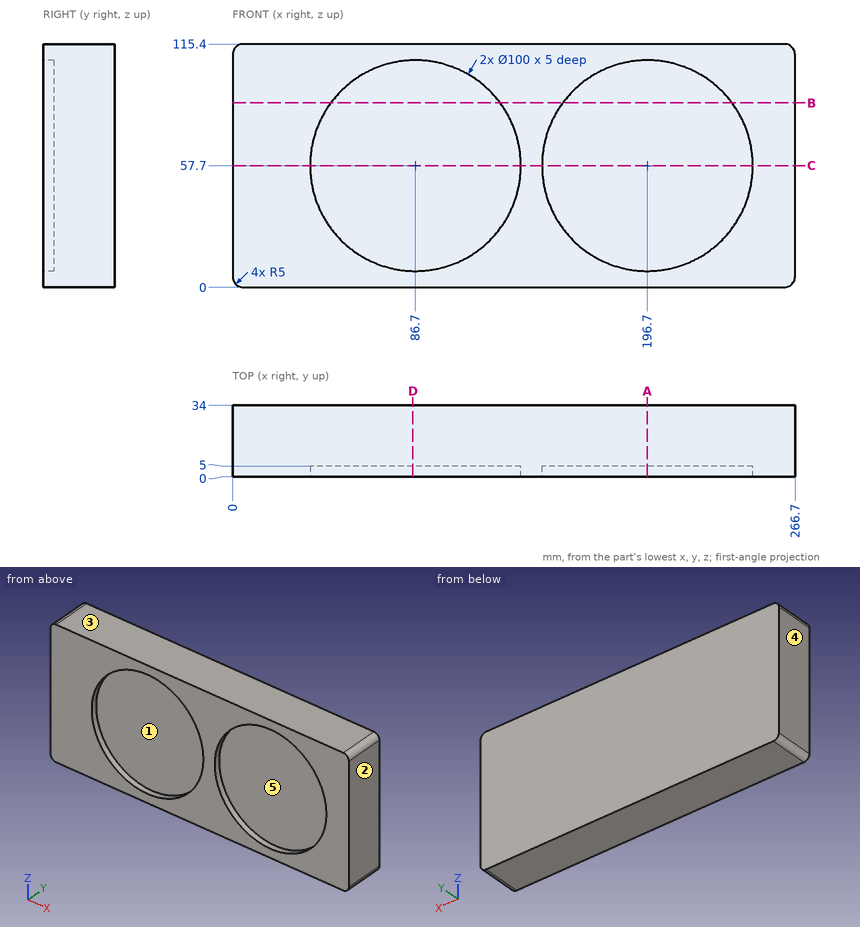
The drawing under review shows one solid part. Ordinate dimensions are in mm from its lowest x, y, z. A direction names the side the tool comes from. Coordinates: 2 decimals unless noted, no trailing zeros. Loops run counter-clockwise (first coordinate to the right, second up) from the corner with the lowest first, then second, coordinate; pieces in that order, holes last. Notation, with made-up numbers: (45, 88.5) - (67, 88.5) arc R23 cw to (67, 102.5) - close; hole circle Ø11 at (26.25, 74.5). An arc over 180 degrees is marked (long way). Return JSON: item names as keys, results as strings.
Item 1: Mouldability with a two-part tool opening along X and no side actions: class the marked faces 3, 4 and 5 as pulls with the +X half, pulls with the -X half, needs draft (parallel to the pull), parting line crosses it, or undercut.
Determined:
{"face 3": "needs draft", "face 4": "pulls with the -X half", "face 5": "undercut"}
Item 2: Insertion check: pin 1 (1 mm diameter, centred on x = 199.5, z = 103, fed in from -Y). The pin has a flat end and moves straight along its axis. Give the tip position at first contact, or say it passes through.
Determined:
{"pin 1": "stops at y = 5"}
Item 3: Take a section at A-A (x = 196.7). Give the boundary of the cut face in (y, z), then the cut area to 3 significant figures.
Determined:
{"outline": "(0, 0) - (34, 0) - (34, 115.4) - (0, 115.4) - (0, 107.7) - (5, 107.7) - (5, 7.7) - (0, 7.7) - close", "area": "3,420 mm2"}
Item 4: For the marked faces 1 and 2, list the 3-axis set-ups (+Z, -Z, +X, -X, +Y, -Y) from which the entire face can be reached by the end or side of a thin tool; tool diameter is ignored.
Determined:
{"face 1": "-Y", "face 2": "+Z, -Z, +X, +Y, -Y"}
Item 5: Take a section at D-D (x = 85.5). Give the boundary of the cut face in (y, z).
Determined:
{"outline": "(0, 0) - (34, 0) - (34, 115.4) - (0, 115.4) - (0, 107.69) - (5, 107.69) - (5, 7.71) - (0, 7.71) - close"}
Item 6: For line 1 (Z direction, x = 86, y = 1); line 2 (X direction, y = 1, z = 57); line 3 (Y direction, x = 54.5, z = 73.5), list the stretches that pass through material, from the lowest coordinate up.
Determined:
{"line 1": "z = 0 to 7.7, 107.7 to 115.4", "line 2": "x = 0 to 36.7, 136.7 to 146.7, 246.7 to 266.7", "line 3": "y = 5 to 34"}
Item 7: Take a section at C-C (z = 57.7). Give the boundary of the cut face in (x, y).
Determined:
{"outline": "(0, 0) - (36.7, 0) - (36.7, 5) - (136.7, 5) - (136.7, 0) - (146.7, 0) - (146.7, 5) - (246.7, 5) - (246.7, 0) - (266.7, 0) - (266.7, 34) - (0, 34) - close"}
Item 8: Take a section at B-B (z = 87.5). Give the boundary of the cut face in (x, y), then the cut area to 3 significant figures.
Determined:
{"outline": "(0, 0) - (46.55, 0) - (46.55, 5) - (126.85, 5) - (126.85, 0) - (156.55, 0) - (156.55, 5) - (236.85, 5) - (236.85, 0) - (266.7, 0) - (266.7, 34) - (0, 34) - close", "area": "8,260 mm2"}
